The figure shows three views and two pictorial views of one solid part (mm, origin at its lowest corner). Answer the questions. A direction names the side the tool comes from. Coordinates: 2 decimals unless noted, no trailing zeros. Write each loop counter-clockwise with the first axis right and the second up, starting at its lowest first coordinate (ties: lowest second). Pieces come first, ordered by that corner, then holes. Notation, with made-up numbers: (81, 78) -> (134, 78) arc R3 ccw to (134, 83) -> close; hole circle Ø4 at (-8, 60.5). An arc over 180 degrees is marked (long way). Use CSV: the item, a comma, the result in double quotes. Start each with the question number.
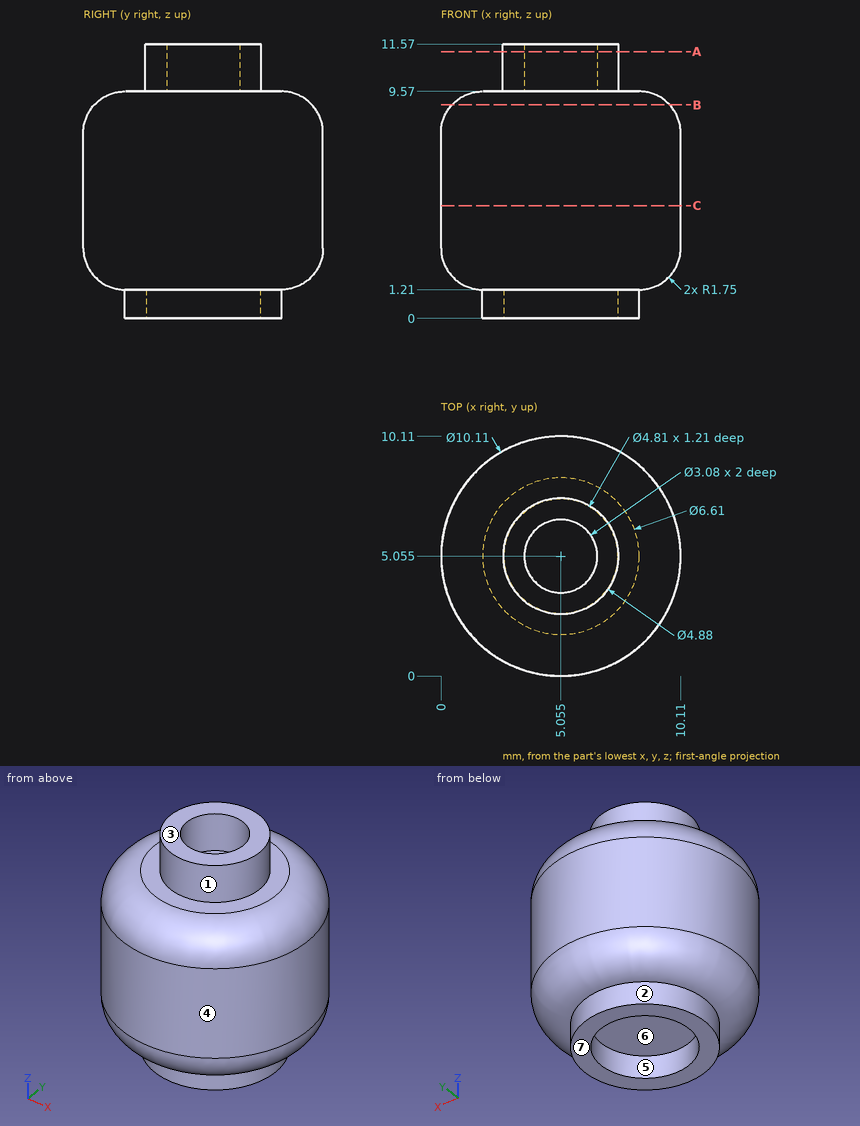
1) The mould has two halves that part along X. Classify the marked faces 4, 5, 6 and 7: pulls with the +X half, pulls with the -X half, needs draft (parallel to the pull), parting line crosses it, or undercut.
2) Section A-A, the plane z = 11.25 is taken. Give the vertices of the cut face in (x, y) (3 decimals).
3) Find the intervals of material crossed by line 1 along Y through (x, z) = (5.25, 4); line 2 along Z through (x, y) = (7, 5.75); line 3 along Z through (x, y) = (6.75, 8), in increasing order.
4) Section C-C, the plane z = 4.75 is taken. Give the vertices of the cut face in (x, y) (3 decimals).
5) Each of these flat-tipped pins is pushed along its axis until it touches: pin 1 (1.4 mm diameter, centred on x = 5, y = 4.5, fed in from -Z); pin 2 (1.5 mm diameter, centred on x = 8.5, y = 4.5, fed in from +Z). Where does it stop, or does it pass through?
6) Section B-B, the plane z = 9 is taken. Give the vertices of the cut face in (x, y) (3 decimals), plus the area to 3 significant figures.
7) Which of the six approach directions +Z, -Z, +X, -X, +Y, -Y give full straight-line access (tool end or side, diameter ignored) to the marked faces 1, 2 and 3?
The answers:
1,face 4,"parting line crosses it"
1,face 5,"undercut"
1,face 6,"undercut"
1,face 7,"needs draft"
2,outline,"circle Ø4.88 at (5.055, 5.055); hole circle Ø3.08 at (5.055, 5.055)"
3,line 1,"y = 0 to 10.11"
3,line 2,"z = 1.21 to 11.57"
3,line 3,"z = 1.21 to 9.57"
4,outline,"circle Ø10.11 at (5.055, 5.055)"
5,pin 1,"stops at z = 1.21"
5,pin 2,"stops at z = 9.57"
6,outline,"circle Ø9.195 at (5.055, 5.055)"
6,area,"66.4 mm^2"
7,face 1,"+Z"
7,face 2,"-Z"
7,face 3,"+Z, +X, -X, +Y, -Y"
